Verification items for the finished model (mm, model axes). Face numbers are marked on the shaded views. Give positions to 0.01 mm unless a question says otherwise; leave off trailing zeros. Loops run counter-clockwise (first coordinate to the right, second up) from the corner with the lowest first, then second, coordinate; pieces in that order, holes last. Notation, with made-up numbers: (-11.5, 20.25) - (26.5, 20.25) arc R15 ccw to (26.5, 25.25) - close; hole circle Ø3 at (50.5, 77.25). An arc over 180 degrees is marked (long way). Answer in a Markdown table with one row per item.
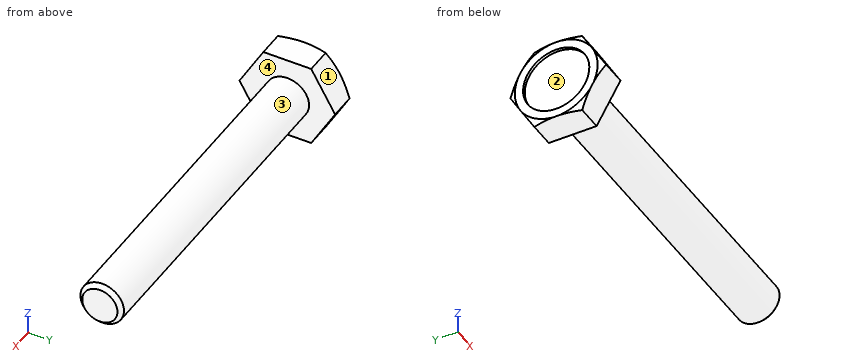
Autodesk Inventor part; units mm, degrees
ref_plane "Work Plane1" through (1.75, 0, 0) normal (0, 0, -1) x (1, 0, 0)
ref_plane "YZ Plane" through (0, 0, 0) normal (1, 0, 0) x (0, 1, 0)
ref_plane "XZ Plane" through (0, 0, 0) normal (0, 1, 0) x (-1, 0, 0)
sketch "Sketch1" plane through (0, 0, 0) normal (0, 0, 1) x (1, 0, 0)
  line L0 (0, 2.0828) -> (31.75, 2.0828)
  line L1 (31.75, 2.0828) -> (31.75, 0)
  line L2 (31.75, 0) -> (0, 0)
  line L3 (0, 0) -> (0, 2.0828)
  line L4 (0, -0.4166) -> (0, 2.4994)
  line L5 (-6.35, 0) -> (38.1, 0)
  dimension "d1" = 4.1656
  dimension "d13" = 31.75
revolve "Body" add sketch "Sketch1" angle 360 about axis through (31.75, 0, 0) along (-1, 0, 0)
sketch "Sketch2" plane through (0, 0, 0) normal (-1, 0, 0) x (0, 0, 1)
  line L0 (0, 4.5754) -> (3.9624, 2.2877)
  line L1 (3.9624, 2.2877) -> (3.9624, -2.2877)
  line L2 (3.9624, -2.2877) -> (0, -4.5754)
  line L3 (0, -4.5754) -> (-3.9624, -2.2877)
  line L4 (-3.9624, -2.2877) -> (-3.9624, 2.2877)
  line L5 (-3.9624, 2.2877) -> (0, 4.5754)
  line L6 (-5.5474, 0) -> (5.5474, 0)
  line L7 (0, 6.4055) -> (0, -6.4055)
  point P0 (0, 0)
  point P1 (0, 0)
  point P2 (0, 0)
  dimension "d8" = 7.9248
extrude "Head" add sketch "Sketch2" along normal blind 2.794
sketch "Sketch3" plane through (-2.794, 0, 0) normal (-1, 0, 0) x (0, 0, 1)
  circle A0 centre (0, 0) radius 3.1699
  point P0 (0, 0)
  dimension "d18" = 6.3398
extrude "Indent" cut sketch "Sketch3" against normal blind 0.2804
sketch "Sketch4" plane through (0, 0, 0) normal (0, 0, 1) x (1, 0, 0)
  line L0 (-2.794, 3.9624) -> (-2.794, 4.5754)
  line L1 (-2.794, 4.5754) -> (-2.4401, 4.5754)
  line L2 (-2.4401, 4.5754) -> (-2.794, 3.9624)
  line L3 (-3.3528, 0) -> (0.5588, 0)
  line L4 (0, 4.5754) -> (-2.794, 4.5754)
  line L5 (-2.794, 2.2877) -> (-2.794, 4.5754)
  dimension "d4" = 30
  dimension "d17" = 7.9248
revolve "Chamfer1" cut sketch "Sketch4" angle 360 about axis through (-10, 0, 0) along (1, 0, 0)
thread "Thread"
chamfer "Chamfer2" distance 0.3975 distance2 0.3976 1 edges at (31.75, -2.0828, 0) measured on face at (31.75, 0.0273, -0.4604)
ref_plane "Work Plane1" through (1.75, 0, 0) normal (0, 0, -1) x (1, 0, 0)
equation "\"d1\" = GD"
equation "\"d13\" = NLG"
equation "\"d8\" = SW"
equation "\"d2\" = KOH - SD"
equation "\"d18\" = KOD2"
equation "\"d4\" = ANG1"
equation "\"d17\" = SW"
equation "\"d9\" = GEL"
equation "\"d5\" = -0.5 * SPD + 0.5 * GD"
equation "\"NLG\" = 31.75"
equation "\"GD\" = NND"
equation "\"BDM\" = NND"
equation "\"KOH\" = 2.794"
equation "\"GEL\" = 26.9875"
equation "\"SW\" = 7.9248"
equation "\"SPD\" = GD1"
equation "\"SD\" = 0"
equation "\"ANG1\" = 30deg"
equation "\"GAL\" = 0.39751"
equation "\"GUL\" = GAL"
equation "\"KOH2\" = 0.1 * KOH"
equation "\"KOD2\" = 0.8 * SW"
equation "\"GD1\" = 3.37058"
equation "\"THREADDIA\" = 4.1656"
equation "\"SDH\" = SW"
equation "\"TOA\" = 30deg"
equation "\"RR\" = 0.04166"
equation "\"NND\" = 4.1656"
equation "\"SW0\" = SW"
equation "\"SD2\" = NND"
equation "\"E0\" = 1.155 * SW"
properties part number "ANSI B18.6.3 - 8-32 UNC - 1.25" material "Steel, Mild"
Q1. Draft check along Y on the marked faces 1, 2, 3 and 4. Enter one of: +Y half, -Y half, draft (parallel to the pull), parting line (faces both ways), or undercut.
Completed:
| item | result |
|---|---|
| face 1 | +Y half |
| face 2 | undercut |
| face 3 | parting line |
| face 4 | draft |
Q2. Thickness scan on line 1 (X direction, y = 2.75, z = -0.75); line 2 (X direction, y = -0.25, z = 3.25); line 3 (Y direction, x = 0.5, z = -0.75). Record the ranges inside material, lowest first.
Completed:
| item | result |
|---|---|
| line 1 | -2.51 to 0 |
| line 2 | -2.79 to 0 |
| line 3 | -1.94 to 1.94 |
Q3. Go/stop test with flat-tipped pins: P1, Ø3, axis at x = 28, z = -1, coming from the -Y side; P2, Ø1.9, axis at y = 1, z = -0.5, coming from the -X side; P3, Ø2, axis at x = 7.5, y = 2.5, coming from the +Z side (3 decimals). Record where each tip stops, or that it passes through.
Completed:
| item | result |
|---|---|
| P1 | y = -2.08 |
| P2 | x = -2.51 |
| P3 | z = 1.445 |
Q4. Sectioned sample at A-A (x = 11). Record the cut outline in (y, z), and give its area (3 significant figures).
Completed:
| item | result |
|---|---|
| outline | circle Ø4.17 at (0, 0) |
| area | 13.6 mm^2 |
